Build history of the part. All positions in model axes, mm. A direction names the side the tool comes from. Round coordinates to 2 decimals unless told otherwise and drop trailing zeros. Write each loop counter-clockwise with the first axis right and the second up, starting at its lowest first coordinate (ties: lowest second). Pieces come first, ordered by that corner, then holes. Notation, with made-up numbers: M -28,60.5 L -12,60.5 A12 cw -12,76.5 Z; hole C -31,35.25 d6. An arc over 180 degrees is marked long. Write item = value, one per line. Start each with the question number.
Q1. Drop flat-ended pins along their axis: P1, Ø5, axis at x = 17.5, y = 0, coming from the -Z side; P2, Ø1, axis at y = 4, z = 7, coming from the -X side; P3, Ø3, axis at x = -14, z = 4.76, coming from the -Y side. Give the stop position or say it passes through.
Q2. Band-saw the part on C-C on y = -19. Write the cut outline in (x, z) (1 decimal), plus the area to 3 significant figures.
Q3. Band-saw the part on D-D on x = 15. Write the cut outline in (y, z) (3 decimals), plus the area to 3 significant figures.
Q4. Band-saw the part on A-A on x = 0. Write the cut outline in (y, z) (3 decimals), plus the area to 3 significant figures.
Q5. Pull direction Z, two halves, no side cores. Call faces 3 (the flat face through (14, -12.395, 5)), 4 (the flat face through (-23.812, -21, 5)), 5 (the flat face through (0, -5, 0)): released by +Z, released by -Z, zero draft, split by the parting line, or undercut.
Q6. Tool access for faces 1 (the cylindrical face through (-1.51, 0.78, 4.7)), 2 (the cylindrical face through (-11.61, -18.81, 4.01)): list every direction of +Z, -Z, +X, -X, +Y, -Y with a clear straight run to the whole face (end or side of a thin tool).
Q7. Band-saw the part on B-B on z = 1. State how many separate pieces and enclosed holes the cut face has, plus the area to 3 significant figures.
Q8. Probe L1, parallel to Y at x = 0, z = 5; L2, parallel to Y at x = -2.5, z = 6; L3, parallel to X at y = -18, z = 7. List the from-to ranges inside material, lowest first.
```python
from build123d import *

# Parameters (mm, degrees)
BOSS_EXTRUDE1_DEPTH       = 9.525
F_10_CLEARANCE_HOLE1_D    = 5.6134
M6X1_0_TAPPED_HOLE1_D     = 5
M6X1_0_TAPPED_HOLE1_DEPTH = 13.0048


with BuildPart() as part:
    # Sketch1 → Boss-Extrude1 (new body)
    with BuildSketch(Plane.XY):
        Polygon((23.8125, -25.4), (23.8125, -15.875), (9.186500373, 25.4), (-6.35, 25.4), (-23.8125, -15.875), (-23.8125, -25.4), align=None)
    extrude(amount=BOSS_EXTRUDE1_DEPTH)

    # #10 Clearance Hole1 (through all)
    with Locations(Plane.XY.offset(9.525)):
        with Locations((0, 20.6375), (0, -1.5875)):
            Hole(F_10_CLEARANCE_HOLE1_D / 2)

    # M6x1.0 Tapped Hole1
    with Locations(Plane(origin=(0, -25.4, 0), x_dir=(-1, 0, 0), z_dir=(0, -1, 0))):
        with Locations((13.9954, -4.7625), (-13.9954, -4.7625)):
            Hole(M6X1_0_TAPPED_HOLE1_D / 2, depth=M6X1_0_TAPPED_HOLE1_DEPTH)


solid = part.part
```
Conclusion:
q1.P1 = 0
q1.P2 = -15.62
q1.P3 = -12.4
q2.outline = M -23.8,0 L 23.8,0 L 23.8,9.5 L -23.8,9.5 Z; hole C -14,4.8 d5; hole C 14,4.8 d5
q2.area = 414 mm^2
q3.outline = M -25.4,0 L 8.994,0 L 8.994,9.525 L -25.4,9.525 L -25.4,7.052 L -12.395,7.052 L -12.395,2.473 L -25.4,2.473 Z
q3.area = 268 mm^2
q4.outline = M -25.4,0 L -4.394,0 L -4.394,9.525 L -25.4,9.525 Z; M 1.219,0 L 17.831,0 L 17.831,9.525 L 1.219,9.525 Z; M 23.444,0 L 25.4,0 L 25.4,9.525 L 23.444,9.525 Z
q4.area = 377 mm^2
q5.face_3 = undercut
q5.face_4 = zero draft
q5.face_5 = released by -Z
q6.face_1 = +Z, -Z
q6.face_2 = -Y
q7.separate_pieces = 1
q7.enclosed_holes = 2
q7.area = 1,710 mm^2
q8.L1 = -25.4 to -4.39, 1.22 to 17.83, 23.44 to 25.4
q8.L2 = -25.4 to -2.86, -0.31 to 19.36, 21.91 to 25.4
q8.L3 = -23.81 to -15.11, -12.88 to 12.88, 15.11 to 23.81
